The figure shows three views and two pictorial views of one solid part (mm, origin at its lowest corner). Answer the questions. A direction names the side the tool comes from. Coordinates: 2 decimals unless noted, no trailing zeros. Order: outer loops, then holes, each group sorted by start corner. A loop starts at its lowest first (then second) coordinate and runs counter-clockwise, first axis right, second up. Notation, with made-up numbers: M -38,59.25 L 11,59.25 A22 ccw 11,72.25 Z; hole C 74,16.25 d9. An arc over 180 degrees is marked long. Answer in a Markdown table with one row per item. Add a question column.
Item 1: Which of the six approach directions +Z, -Z, +X, -X, +Y, -Y give full straight-line access (tool end or side, diameter ignored) to the marked faces 1 and 2?
Item 2: The part is cut by section A-A (x = 3.75). Write down the section's boundary in (y, z), then the cut area to 3 significant figures.
Item 3: The part is cut by section B-B (z = 0.4). Write down the section's boundary in (x, y), then the cut area to 3 significant figures.
Item 4: The part is cut by section D-D (x = 7.5). Write down the section's boundary in (y, z), then the cut area to 3 significant figures.
Item 5: Consider line 1 (Y direction, x = 7.5, z = 1.35); line 2 (Y direction, x = 3.75, z = 1.05); line 3 (X direction, y = 3.25, z = 0.15). Determine where each line is inside the solid, lowest interval first. Write a range as from..to.
Item 6: The part is cut by section C-C (y = 2.5). Write down the section's boundary in (x, z), then the cut area to 3 significant figures.
Item 7: A flat-ended cylindrical pin translates along its axis: pin 1 Ø5 at (x, y) = (3.75, 2.5) entering from -Z. Find the tip coordinate at first contact, or state that the pin passes through.
Item 8: The mould has two halves that part along Y. Classify the marked faces 3, 4, 5 and 6: released by +Y, released by -Y, zero draft, split by the parting line, or undercut.
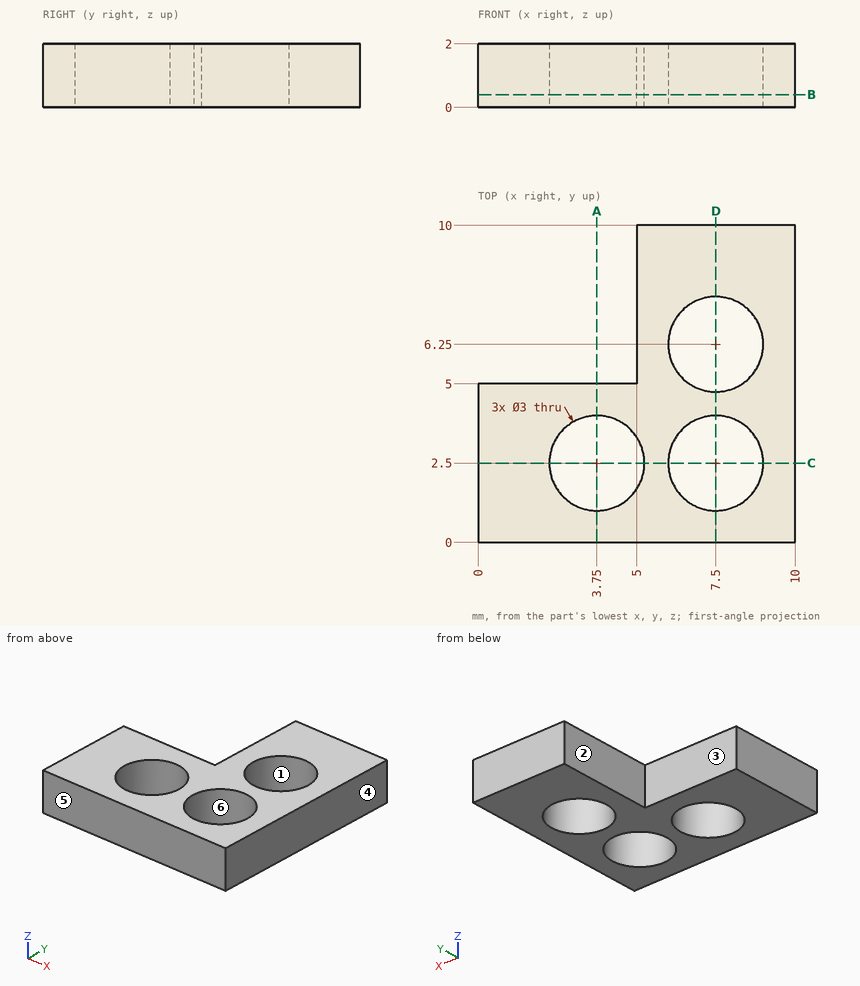
Reply:
| question | item | result |
|---|---|---|
| 1 | face 1 | +Z, -Z |
| 1 | face 2 | +Z, -Z, -X, +Y |
| 2 | outline | M 0,0 L 1,0 L 1,2 L 0,2 Z; M 4,0 L 5,0 L 5,2 L 4,2 Z |
| 2 | area | 4.00 mm2 |
| 3 | outline | M 0,0 L 10,0 L 10,10 L 5,10 L 5,5 L 0,5 Z; hole C 3.75,2.5 d3; hole C 7.5,2.5 d3; hole C 7.5,6.25 d3 |
| 3 | area | 53.8 mm2 |
| 4 | outline | M 0,0 L 1,0 L 1,2 L 0,2 Z; M 4,0 L 4.75,0 L 4.75,2 L 4,2 Z; M 7.75,0 L 10,0 L 10,2 L 7.75,2 Z |
| 4 | area | 8.00 mm2 |
| 5 | line 1 | y = 0..1, 4..4.75, 7.75..10 |
| 5 | line 2 | y = 0..1, 4..5 |
| 5 | line 3 | x = 0..2.45, 5.05..6.2, 8.8..10 |
| 6 | outline | M 0,0 L 2.25,0 L 2.25,2 L 0,2 Z; M 5.25,0 L 6,0 L 6,2 L 5.25,2 Z; M 9,0 L 10,0 L 10,2 L 9,2 Z |
| 6 | area | 8.00 mm2 |
| 7 | pin 1 | stops at z = 0 |
| 8 | face 3 | released by +Y |
| 8 | face 4 | zero draft |
| 8 | face 5 | released by -Y |
| 8 | face 6 | undercut |
